Verification items for the finished model (mm, model axes). A direction names the side the tool comes from. Give positions to 0.01 mm unless a question says otherwise; leave off trailing zeros. Loops run counter-clockwise (first coordinate to the right, second up) from the corner with the lowest first, then second, coordinate; pieces in that order, holes last. Notation, with made-up numbers: (35.5, 71) - (92.5, 71) arc R10 ccw to (92.5, 76) - close; hole circle Ø1 at (62, -31). An arc over 180 degrees is marked (long way). One line per item, written item: value. Start each with the question number.
1. Gauge pin test, flat ends, axial feed: pin 1 (3 mm diameter, centred on x = 9, y = 2.5, fed in from +Z); pin 2 (2.5 mm diameter, centred on y = 0, z = 5, fed in from +X); pin 3 (2 mm diameter, centred on x = 12.5, y = -3.5, fed in from +Z). Record the tip position at first contact, or that the pin passes through.
2. Sectioned sample at C-C (x = 21.5). Record the cut outline in (y, z), plus the area to 3 significant figures.
3. Access from +Z, -Z, +X, -X, +Y, -Y to the whole of each face (thin tool, end or side, straight path). Record for faces 5 (the flat face through (40, 0, 1)), 6 (the flat face through (20, -4, 0)), 7 (the flat face through (19.7, 5, 8.5)).
4. Sectioned sample at D-D (z = 8.5). Record the cut outline in (x, y), plus the area to 3 significant figures.
5. Scan lines: L1, parallel to Z at x = -1.1, y = 0; L2, parallel to Y at x = -1.05, z = 5; L3, parallel to Y at x = 16, z = 8.25. Record each from-to range of solid material in increasing order. Write a range as [from, to].
6. Sectioned sample at A-A (y = 0). Record the cut outline in (x, z).
7. Mould release check, pull along Y, two halves, no side actions. Record for faces 1 (the cylindrical face through (19.72, -3.557, 5.458)), 2 (the flat face through (19, 6, 4)), 3 (the flat face through (19, 0, -1)), 4 (the cylindrical face through (19.72, 3.557, 5.542)): pulls with the +Y half, pulls with the -Y half, needs draft (parallel to the pull), parting line crosses it, or undercut.
8. Sectioned sample at B-B (z = 5). Record the cut outline in (x, y), plus the area to 3 significant figures.
from build123d import *

# Parameters (mm, degrees)
PAD_DEPTH    = 40
SKETCH001_W  = 12
SKETCH001_H  = 10
SKETCH001_R  = 1.6
PAD001_DEPTH = 2


with BuildPart() as part:
    # Sketch → Pad (new body)
    with BuildSketch(Plane.YZ):
        with BuildLine():
            Line((-5, 8), (-5, 9))
            Line((-5, 9), (-6, 9))
            Line((-6, 9), (-6, -1))
            Line((-6, -1), (6, -1))
            Line((6, -1), (6, 9))
            Line((6, 9), (5, 9))
            Line((5, 9), (5, 8))
            ThreePointArc((5, 8), (3.556624, 5.5), (5, 3))
            Line((5, 3), (5, 0))
            Line((5, 0), (2.5, 0))
            ThreePointArc((2.5, 0), (0, 1.443376), (-2.5, 0))
            Line((-2.5, 0), (-5, 0))
            Line((-5, 0), (-5, 3))
            ThreePointArc((-5, 3), (-3.556624, 5.5), (-5, 8))
        make_face()
    extrude(amount=PAD_DEPTH)

    # Sketch001 (on Face15 of Pad) → Pad001 (join)
    with BuildSketch(Plane(origin=(0, 0, 0), x_dir=(0, 1, 0), z_dir=(-1, 0, 0))):
        with Locations((0, -4)):
            Rectangle(SKETCH001_W, SKETCH001_H)
        with Locations((0, -5)):
            Circle(SKETCH001_R, mode=Mode.SUBTRACT)
    extrude(amount=PAD001_DEPTH)


solid = part.part
Results are:
1. pin 1: stops at z = 7.04
1. pin 2: passes through
1. pin 3: stops at z = 7.63
2. outline: (-6, -1) - (6, -1) - (6, 9) - (5, 9) - (5, 8) arc R2.89 ccw to (5, 3) - (5, 0) - (2.5, 0) arc R2.89 ccw to (-2.5, 0) - (-5, 0) - (-5, 3) arc R2.89 ccw to (-5, 8) - (-5, 9) - (-6, 9) - close
2. area: 45.4 mm^2
3. face 5: +Z, -Z, +X, +Y, -Y
3. face 6: +X
3. face 7: +Z, +X
4. outline: (-2, -6) - (40, -6) - (40, -5) - (0, -5) - (0, 5) - (40, 5) - (40, 6) - (-2, 6) - close
4. area: 104 mm^2
5. L1: z = [-1, 3.4], [6.6, 9]
5. L2: y = [-6, -1.6], [1.6, 6]
5. L3: y = [-6, -5], [5, 6]
6. outline: (-2, -1) - (40, -1) - (40, 1.44) - (0, 1.44) - (0, 3.4) - (-2, 3.4) - close; (-2, 6.6) - (0, 6.6) - (0, 9) - (-2, 9) - close
7. face 1: undercut
7. face 2: pulls with the +Y half
7. face 3: needs draft
7. face 4: undercut
8. outline: (-2, -6) - (40, -6) - (40, -3.6) - (0, -3.6) - (0, -1.6) - (-2, -1.6) - close; (-2, 1.6) - (0, 1.6) - (0, 3.6) - (40, 3.6) - (40, 6) - (-2, 6) - close
8. area: 210 mm^2
